from build123d import *

# Parameters (mm, degrees)
SKETCH1_R           = 1.5
BOSS_EXTRUDE1_DEPTH = 5


with BuildPart() as part:
    # Sketch1 → Boss-Extrude1 (new body)
    with BuildSketch(Plane(origin=(0, 0, 0), x_dir=(1, 0, 0), z_dir=(0, 1, 0))):
        with BuildLine():
            ThreePointArc((30.05067828, -1.98711795), (17.911907525, 1.279041193), (7.386236134, 8.151289209))
            ThreePointArc((7.386236134, 8.151289209), (-8.425357061, 7.07201233), (-6.747627634, -8.68731957))
            ThreePointArc((-6.747627634, -8.68731957), (24.327807705, -28.522008688), (58.515872209, -42.315986336))
            ThreePointArc((58.515872209, -42.315986336), (69.43935161, -43.996070724), (80.405631289, -42.622827932))
            ThreePointArc((80.405631289, -42.622827932), (183.01994094, -26.16258262), (286.820423183, -31.271017511))
            ThreePointArc((286.820423183, -31.271017511), (299.326255976, -22.347352445), (290.71394184, -9.625100394))
            ThreePointArc((290.71394184, -9.625100394), (202.127360194, -0.420820539), (113.463070734, -8.843705436))
            ThreePointArc((113.463070734, -8.843705436), (96.019370903, -7.044766711), (82.561456398, 4.198159132))
            ThreePointArc((82.561456398, 4.198159132), (72.12928734, 10.848102082), (60.248711806, 7.397911149))
            ThreePointArc((60.248711806, 7.397911149), (46.116503766, -0.405485841), (30.05067828, -1.98711795))
        make_face()
        with Locations((130, -19)):
            Circle(SKETCH1_R, mode=Mode.SUBTRACT)
        with Locations((250, -17)):
            Circle(SKETCH1_R, mode=Mode.SUBTRACT)
        with Locations((288.5, -20.4)):
            Circle(SKETCH1_R, mode=Mode.SUBTRACT)
        with Locations((70, -4)):
            Circle(SKETCH1_R, mode=Mode.SUBTRACT)
        Circle(SKETCH1_R, mode=Mode.SUBTRACT)
    extrude(amount=BOSS_EXTRUDE1_DEPTH)


solid = part.part
Could you check a few things on this model? Use its own coordinates, in mm. Coordinates: 2 decimals unless noted, no trailing zeros. Write each loop counter-clockwise with the first axis right and the second up, starting at its lowest first coordinate (ties: lowest second). Pieces come first, ordered by that corner, then holes. Notation, with made-up numbers: (13, 64.5) - (35, 64.5) arc R19 ccw to (35, 79.5) - close; hole circle Ø10 at (73.5, 14.5). An arc over 180 degrees is marked (long way). Write item = value, one per line.
1) Suppose I cut it at C-C on z = 38. Please give me the cut outline in (x, y).
Result set:
outline = (45.71, 0) - (98.97, 0) - (98.97, 5) - (45.71, 5) - close
2) Will these pins go through, and if not, where does the flat tip stop? pin 1 Ø2 at (x, y) = (41.5, 3.5) entering from -Z; pin 2 Ø2.5 at (x, z) = (130, 19) entering from +Y; pin 3 Ø2 at (y, z) = (4.5, 10) entering from -X.
Result set:
pin_1 = 1.35
pin_2 = through
pin_3 = -6.34
3) Please list where these lines run through material, in increasing order: line 1 (Z direction, x = 288.5, y = 2.9); line 2 (X direction, y = 0.45, z = -7.5); line 3 (Z direction, x = 225.5, y = 3.8). Write a range as [from, to].
Result set:
line_1 = [9.18, 18.9], [21.9, 31.4]
line_2 = [-8.05, 8.12], [60.37, 79.63]
line_3 = [1.13, 25.63]
4) Suppose I cut it at A-A on y = 3.15. Please give me the cut outline in (x, z).
Result set:
outline = (-6.75, 8.69) arc R11 ccw (long way) to (7.39, -8.15) arc R40 cw to (60.25, -7.4) arc R15 ccw to (82.56, -4.2) arc R30 cw to (113.46, 8.84) arc R450 ccw to (290.71, 9.63) arc R11 ccw to (286.82, 31.27) arc R500 cw to (80.41, 42.62) arc R40 ccw to (58.52, 42.32) arc R200 ccw to start; hole circle Ø3 at (0, 0); hole circle Ø3 at (70, 4); hole circle Ø3 at (130, 19); hole circle Ø3 at (250, 17); hole circle Ø3 at (288.5, 20.4)
5) Suppose I cut it at B-B on x = 49.5. Please give me the cut outline in (y, z).
Result set:
outline = (0, -0.82) - (5, -0.82) - (5, 39.38) - (0, 39.38) - close
6) We'd pull the mould along Y, two halves only. Please class faces 1 (the flat face through (142, 5, 16)), 2 (the flat face through (142, 0, 16)), 3 (the cylindrical face through (96.25, 2.46, 7.14)): +Y half, -Y half, draft (parallel to the pull), parting line (faces both ways), or undercut.
Result set:
face_1 = +Y half
face_2 = -Y half
face_3 = draft
